Could you check a few things on this drawing? It's one solid part, dimensions in mm from its lowest x, y, z. Give positions to 0.01 mm unless a question says otherwise; leave off trailing zeros. Order: outer loops, then holes, each group sorted by start corner. A loop starts at its lowest first (then second) coordinate and runs counter-clockwise, first axis right, second up.
Item 1: I want a section at B-B, the plane z = 1.25. Count the separate pieces of the cut face and the enclosed holes in it, then the cut area to 3 significant figures.
Item 2: If I drill on line 1 along Y through (x, z) = (38.1, 3.5); line 2 along Y through (x, z) = (32.5, 1.25) (1 decimal); line 3 along X through (y, z) = (4.5, 3.5) (1 decimal), over which ranges is the centre line in solid material (lowest first)?
Item 3: I want a section at C-C, the plane y = 62.5. Write out the boundary of the cut face in (x, z).
Item 4: I'm going to push flat-ended pins straight in: pin 1 Ø10 at (x, y) = (38.1, 26.02) entering from +Z; pin 2 Ø3 at (x, z) = (60, 1) entering from +Y (1 decimal). Where does each tip first touch, or does it pass through?
Item 5: If we mould it in two halves opening along Y, with no side actions, what happens to the marked faces 1, 2 and 3? For each: +Y half, -Y half, draft (parallel to the pull), parting line (faces both ways), or undercut.
Item 6: I want a section at A-A, the plane x = 38.1. Write out the boundary of the cut face in (y, z).
Item 7: I want a section at D-D, the plane x = 6. Write out the boundary of the cut face in (y, z).
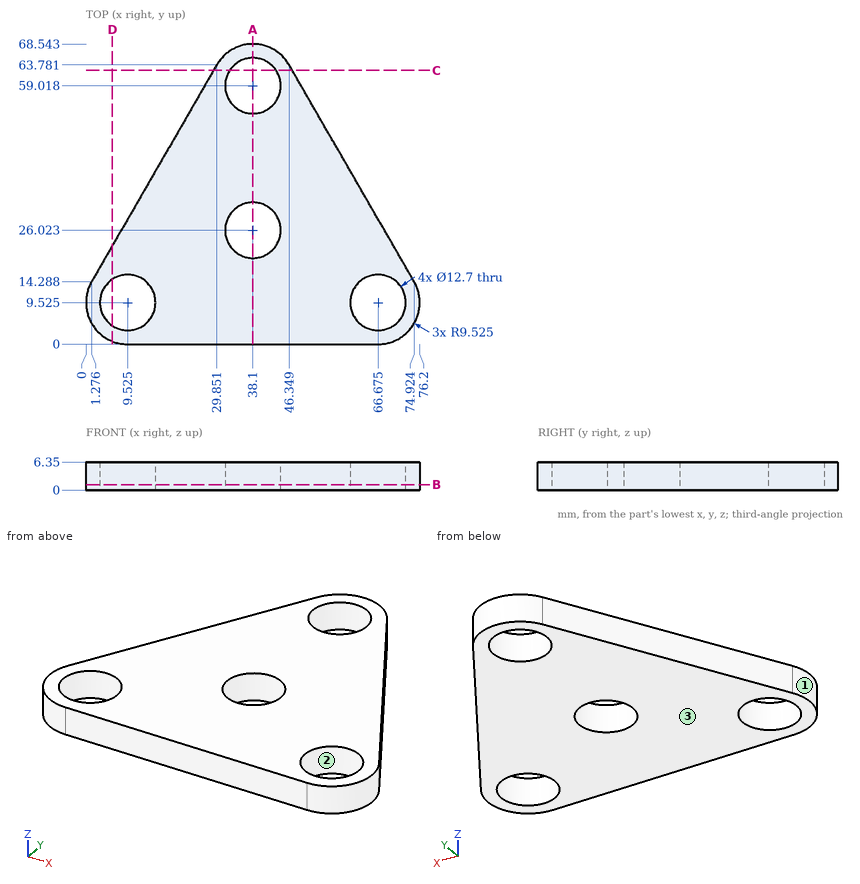
Results list:
1. separate pieces: 1
1. enclosed holes: 4
1. area: 2,830 mm2
2. line 1: y = 0 to 19.67, 32.37 to 52.67, 65.37 to 68.54
2. line 2: y = 0 to 23, 29 to 56, 62 to 66.7
2. line 3: x = 1.4 to 5.6, 13.4 to 62.8, 70.6 to 74.8
3. outline: (29.11, 0) - (32.79, 0) - (32.79, 6.35) - (29.11, 6.35) - close; (43.41, 0) - (47.09, 0) - (47.09, 6.35) - (43.41, 6.35) - close
4. pin 1: passes through
4. pin 2: stops at y = 42.7
5. face 1: parting line
5. face 2: undercut
5. face 3: draft
6. outline: (0, 0) - (19.67, 0) - (19.67, 6.35) - (0, 6.35) - close; (32.37, 0) - (52.67, 0) - (52.67, 6.35) - (32.37, 6.35) - close; (65.37, 0) - (68.54, 0) - (68.54, 6.35) - (65.37, 6.35) - close
7. outline: (0.68, 0) - (4.24, 0) - (4.24, 6.35) - (0.68, 6.35) - close; (14.81, 0) - (22.47, 0) - (22.47, 6.35) - (14.81, 6.35) - close
